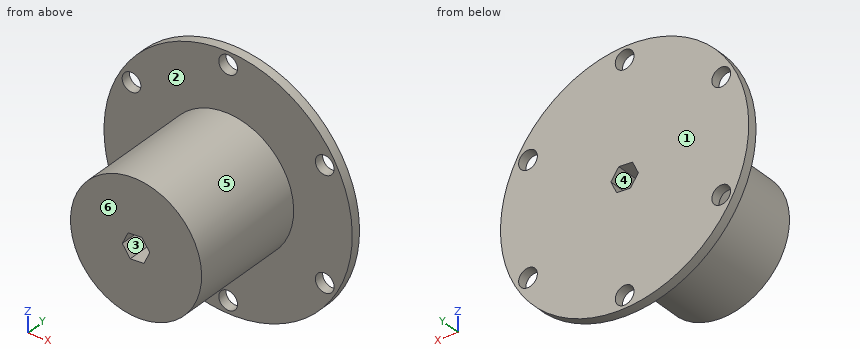
from build123d import *

# Parameters (mm, degrees)
SKETCH1_R           = 14
BOSS_EXTRUDE1_DEPTH = 25.3
SKETCH2_R           = 26.5
BOSS_EXTRUDE2_DEPTH = 2
SKETCH3_R           = 2
CUT_EXTRUDE1_DEPTH  = 32


with BuildPart() as part:
    # Sketch1 → Boss-Extrude1 (new body)
    with BuildSketch(Plane(origin=(0, 0, 0), x_dir=(1, 0, 0), z_dir=(0, 1, 0))):
        with Locations(Location((0, 0, 0), (0, 0, 270))):
            Circle(SKETCH1_R)
    extrude(amount=BOSS_EXTRUDE1_DEPTH)

    # Sketch2 → Boss-Extrude2 (add)
    with BuildSketch(Plane(origin=(0, 25.3, 0), x_dir=(1, 0, 0), z_dir=(0, 1, 0))):
        with Locations(Location((0, 0, 0), (0, 0, 270))):
            Circle(SKETCH2_R)
    extrude(amount=BOSS_EXTRUDE2_DEPTH)

    # Sketch3 → Cut-Extrude1 (cut)
    with BuildSketch(Plane(origin=(0, 27.3, 0), x_dir=(1, 0, 0), z_dir=(0, 1, 0))):
        with Locations(Location((0, 23.815, 0), (0, 0, 270))):
            Circle(SKETCH3_R)
        with Locations(Location((20.624394991, 11.9075, 0), (0, 0, 270))):
            Circle(SKETCH3_R)
        with Locations(Location((20.624394991, -11.9075, 0), (0, 0, 270))):
            Circle(SKETCH3_R)
        with Locations(Location((0, -23.815, 0), (0, 0, 270))):
            Circle(SKETCH3_R)
        with Locations(Location((-20.624394991, -11.9075, 0), (0, 0, 270))):
            Circle(SKETCH3_R)
        with Locations(Location((-20.624394991, 11.9075, 0), (0, 0, 270))):
            Circle(SKETCH3_R)
        Polygon((1.234520104, -2.673192869), (2.932312985, -0.267470663), (1.697792881, 2.405722206), (-1.234520104, 2.673192869), (-2.932312985, 0.267470663), (-1.697792881, -2.405722206), align=None)
    extrude(amount=-CUT_EXTRUDE1_DEPTH, mode=Mode.SUBTRACT)


solid = part.part
The listing builds one solid part. Answer for the finished solid, in the listing's coordinates (mm). Face numbers are marked on the shaded views. A direction names the side the tool comes from. Give positions to 0.01 mm unless a question says otherwise; leave off trailing zeros. Write each loop counter-clockwise with the first axis right and the second up, starting at its lowest first coordinate (ties: lowest second). Pieces come first, ordered by that corner, then holes. Notation, with made-up numbers: (80.25, 70) - (108.25, 70) arc R23 cw to (108.25, 102) - close; hole circle Ø2 at (-18.75, -18). An arc over 180 degrees is marked (long way). One line per question, with ' | ' between items. Start each with the question number.
1. For the marked faces 1, 2 and 3, determine the directions among +Z, -Z, +X, -X, +Y, -Y from which every point of the face is accessible in a straight line to the end or side of a thin tool.
2. Determine the mould class of the marked faces 4, 5 and 6 for opening direction Z: +Z half, -Z half, draft (parallel to the pull), parting line (faces both ways), or undercut.
3. Section D-D, the plane x = -8 is taken. Determine the outline of the cut face in (y, z), then the cut area to 3 significant figures.
4. Straight lines are drawn through the part: line 1 (Z direction, x = 1, y = 18.25); line 2 (Z direction, x = 2, y = 15); line 3 (Y direction, x = -13.5, z = 7). For each, find the intervals that lie inside material, in ascending order.
5. Section B-B, the plane x = 0 is taken. Determine the outline of the cut face in (y, z) (3 decimals), then the cut area to 3 significant figures.
6. Section A-A, the plane y = 11 is taken. Determine the outline of the cut face in (x, z), then the cut area to 3 significant figures.
7. Section C-C, the plane z = -6 is taken. Determine the outline of the cut face in (x, y).
8. Given P1, Ø4.5, axis at x = 20.62, z = 11.91, coming from the -Y side; P2, Ø1.5, axis at y = 17.5, z = -6.5, coming from the +X side; P3, Ø4, axis at x = 0.5, y = 14.5, coming from the +Z side, each flat-ended and moving along its own axis, determine where each tip first touches the part or whether it passes through.
Result:
1) face 1: +Z, -Z, +X, -X, +Y | face 2: -Y | face 3: +Y, -Y
2) face 4: undercut | face 5: parting line | face 6: draft
3) outline: (0, -11.49) - (25.3, -11.49) - (25.3, -25.26) - (27.3, -25.26) - (27.3, 25.26) - (25.3, 25.26) - (25.3, 11.49) - (0, 11.49) - close | area: 682 mm2
4) line 1: z = -13.96 to -2.47, 2.65 to 13.96 | line 2: z = -13.86 to -1.75, 1.59 to 13.86 | line 3: y = 25.3 to 27.3
5) outline: (0, -14) - (25.3, -14) - (25.3, -21.815) - (27.3, -21.815) - (27.3, -2.561) - (0, -2.561) - close; (0, 2.561) - (27.3, 2.561) - (27.3, 21.815) - (25.3, 21.815) - (25.3, 14) - (0, 14) - close; (25.3, -26.5) - (27.3, -26.5) - (27.3, -25.815) - (25.3, -25.815) - close; (25.3, 25.815) - (27.3, 25.815) - (27.3, 26.5) - (25.3, 26.5) - close | area: 659 mm2
6) outline: circle Ø28 at (0, 0); hole (-2.93, -0.27) - (-1.23, -2.67) - (1.7, -2.41) - (2.93, 0.27) - (1.23, 2.67) - (-1.7, 2.41) - close | area: 593 mm2
7) outline: (-25.81, 25.3) - (-12.65, 25.3) - (-12.65, 0) - (12.65, 0) - (12.65, 25.3) - (25.81, 25.3) - (25.81, 27.3) - (-25.81, 27.3) - close
8) P1: stops at y = 25.3 | P2: stops at x = 12.76 | P3: stops at z = 14
